Part model, mm, in its own coordinate system. Face numbers are marked on the shaded views. A direction names the side the tool comes from. Give positions to 0.01 mm unless a question says otherwise; leave off trailing zeros. Write each loop counter-clockwise with the first axis right and the second up, starting at its lowest first coordinate (ties: lowest second). Pieces come first, ordered by that corner, then holes. Notation, with made-up numbers: M 75,3 L 134,3 A17 cw 134,28 Z; hole C 74.25,6.25 d11. An arc over 180 degrees is marked long. Answer as CSV lines item,"result". Start each with the question number.
Item 1: Band-saw the part on A-A, the plane y = 0. List the corners of the cut face in (x, z).
Item 2: Wall check: L1, parallel to Z at x = 11.5, y = 12; L2, parallel to Z at x = -7, y = -1.5; L3, parallel to Y at x = -0.5, z = 46 (3 decimals). Give the ranges that are in metal, low to high. Write a range as from..to.
Item 3: Band-saw the part on D-D, the plane z = 38. List the corners of the cut face in (x, y).
Item 4: 3-axis set-ups, long thin cutter, end or side, ignore diameter. For the marked faces 5 and 6: which of +Z, -Z, +X, -X, +Y, -Y reach the whole face in a straight line?
Item 5: Pin check, flat tips, straight feed: pin 1 (15 mm diameter, centred on x = 5, y = 0.5, fed in from -Z); pin 2 (10 mm diameter, centred on x = -14.5, y = -15, fed in from -Z); pin 3 (3 mm diameter, centred on y = -4, z = 14.5, fed in from +X); pin 4 (6 mm diameter, centred on x = -11, z = 42, fed in from +Y). Stop position of each tip, or through.
Item 6: Two-plate mould, pull along Z, no slides. Class the marked faces 1, 2, 3 and 4: +Z half, -Z half, draft (parallel to the pull), parting line (faces both ways), or undercut.
Item 7: Band-saw the part on B-B, the plane z = 22. List the corners of the cut face in (x, y).
Item 8: Band-saw the part on C-C, the plane x = -5. List the corners of the cut face in (y, z), then the cut area to 3 significant figures.
Autodesk Inventor part; units mm, degrees
ref_plane "YZ Plane" through (0, 0, 0) normal (1, 0, 0) x (0, 1, 0)
ref_plane "XZ Plane" through (0, 0, 0) normal (0, 1, 0) x (-1, 0, 0)
ref_plane "XY Plane" through (0, 0, 0) normal (0, 0, 1) x (1, 0, 0)
sketch "Sketch1" plane through (0, 0, 0) normal (0, 0, 1) x (1, 0, 0)
  circle A0 centre (0, 0) radius 6
  dimension "d0" = 12
extrude "Extrusion1" add sketch "Sketch1" along normal blind 35
thread "Thread1"
sketch "Sketch2" plane through (0, 0, 35) normal (0, 0, 1) x (1, 0, 0)
  circle A0 centre (0, 0) radius 7.5
  dimension "d5" = 15
extrude "Extrusion2" add sketch "Sketch2" along normal blind 5
sketch "Sketch3" plane through (0, 0, 40) normal (0, 0, 1) x (1, 0, 0)
  circle A0 centre (0, 0) radius 25
  dimension "d8" = 50
extrude "Extrusion3" add sketch "Sketch3" along normal blind 10
sketch "Sketch4" plane through (0, 0, 35) normal (0, 0, -1) x (-1, 0, 0)
  line L0 (0, 6.9282) -> (6, 3.4641)
  line L1 (6, 3.4641) -> (6, -3.4641)
  line L2 (6, -3.4641) -> (0, -6.9282)
  line L3 (0, -6.9282) -> (-6, -3.4641)
  line L4 (-6, -3.4641) -> (-6, 3.4641)
  line L5 (-6, 3.4641) -> (0, 6.9282)
  line L6 (0, 9.2376) -> (8, 4.6188)
  line L7 (8, 4.6188) -> (8, -4.6188)
  line L8 (8, -4.6188) -> (0, -9.2376)
  line L9 (0, -9.2376) -> (-8, -4.6188)
  line L10 (-8, -4.6188) -> (-8, 4.6188)
  line L11 (-8, 4.6188) -> (0, 9.2376)
  point P0 (0, 0)
  point P1 (0, 0)
  point P2 (0, 0)
  dimension "d11" = 6
  dimension "d12" = 8
extrude "Extrusion4" add sketch "Sketch4" along normal blind 5 contours L0 L1 L2 L3 L4 L5 | L6 L7 L8 L9 L10 L11
properties part number "ChanBangTai"
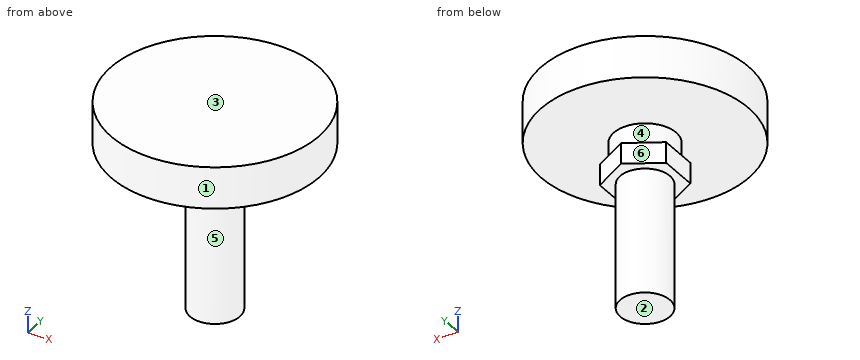
Output:
1,outline,"M -25,40 L -7.5,40 L -7.5,35 L -8,35 L -8,30 L -6,30 L -6,0 L 6,0 L 6,30 L 8,30 L 8,35 L 7.5,35 L 7.5,40 L 25,40 L 25,50 L -25,50 Z"
2,L1,"40..50"
2,L2,"30..50"
2,L3,"-24.995..24.995"
3,outline,"C 0,0 d15"
4,face 5,"-Z"
4,face 6,"-Z, -X, +Y"
5,pin 1,"z = 0"
5,pin 2,"z = 40"
5,pin 3,"x = 5.45"
5,pin 4,"y = 23.69"
6,face 1,"draft"
6,face 2,"-Z half"
6,face 3,"+Z half"
6,face 4,"undercut"
7,outline,"C 0,0 d12"
8,outline,"M -24.49,40 L -5.59,40 L -5.59,35 L -6.35,35 L -6.35,30 L -3.32,30 L -3.32,0 L 3.32,0 L 3.32,30 L 6.35,30 L 6.35,35 L 5.59,35 L 5.59,40 L 24.49,40 L 24.49,50 L -24.49,50 Z"
8,area,"808 mm²"
